Verification items for the finished model (mm, model axes). Face numbers are marked on the shaded views. Coordinates: 2 decimals unless noted, no trailing zeros. Order: outer loops, then holes, each group sorted by start corner. A loop starts at its lowest first (then second) coordinate and runs counter-clockwise, first axis right, second up.
Q1. Draft check along Z on the marked faces 1, 2, 3 and 4. Enter one of: pulls with the +Z half, pulls with the -Z half, needs draft (parallel to the pull), parting line crosses it, or undercut.
Q2. Cross-section at B-B, the plane y = -66.5. Record the boundary of the cut face in (x, z), and give its area (3 significant figures).
Q3. Cross-section at D-D, the plane z = 32. Record the boundary of the cut face in (x, y).
Q4. Cross-section at C-C, the plane x = -15.25. Record the boundary of the cut face in (y, z), and give its area (3 significant figures).
Q5. Depth check by flat-ended pin: P1, Ø3, axis at y = -26.5, z = -15, coming from the +X side; P2, Ø5.5, axis at x = -9.22, y = -50.8, coming from the -Z side. Enter the tip coordinate at first touch or a pass-through.
Q6. Thickness scan on line 1 (Z direction, x = -18.25, y = -7); line 2 (X direction, y = -39.5, z = 41); line 3 (X direction, y = -50, z = -34). Record the ranges inside material, lowest first.
Q7. Cross-section at A-A, the plane y = -50.8. Record the boundary of the cut face in (x, z).
from build123d import *

# Parameters (mm, degrees)
F1_DEPTH = 88.9
F2_R     = 3.175
F3_DEPTH = 101.6
F5_DEPTH = 3.175


with BuildPart() as f1:
    # F0 (on Front) → F1 (new body)
    with BuildSketch(Plane.XZ):
        Polygon((3.47705, 44.675883), (-21.92295, 44.675883), (-21.92295, -35.715117), (3.47705, -35.715117), (3.47705, -32.540117), (-18.74795, -32.540117), (-18.74795, 41.500883), (3.47705, 41.500883), align=None)
    extrude(amount=F1_DEPTH)

    # F2 (on face) → F3 (cut)
    with BuildSketch(Plane.XY.offset(44.675883)):
        with Locations((-9.22295, -76.2)):
            Circle(F2_R)
        with Locations((-9.22295, -50.8)):
            Circle(F2_R)
        with Locations((-9.22295, -25.4)):
            Circle(F2_R)
        with Locations((-9.22295, 0)):
            Circle(F2_R)
        with Locations((-34.62295, -76.2)):
            Circle(F2_R)
        with Locations((-34.62295, -50.8)):
            Circle(F2_R)
        with Locations((-34.62295, -25.4)):
            Circle(F2_R)
        with Locations((-34.62295, 0)):
            Circle(F2_R)
    extrude(amount=-F3_DEPTH, mode=Mode.SUBTRACT)

    # F4 (on face) → F5 (cut)
    with BuildSketch(Plane.XY.offset(44.675883)):
        with BuildLine():
            Line((-17.16045, 0), (3.47705, -11.915066))
            Line((3.47705, -11.915066), (3.47705, 0))
            Line((3.47705, 0), (-6.04795, 0))
            ThreePointArc((-6.04795, 0), (-9.22295, -3.175), (-12.39795, 0))
            Line((-12.39795, 0), (-17.16045, 0))
        make_face()
        Polygon((3.47705, -76.521958), (-17.962348, -88.9), (3.47705, -88.9), align=None)
    extrude(amount=-F5_DEPTH, mode=Mode.SUBTRACT)


solid = f1.part
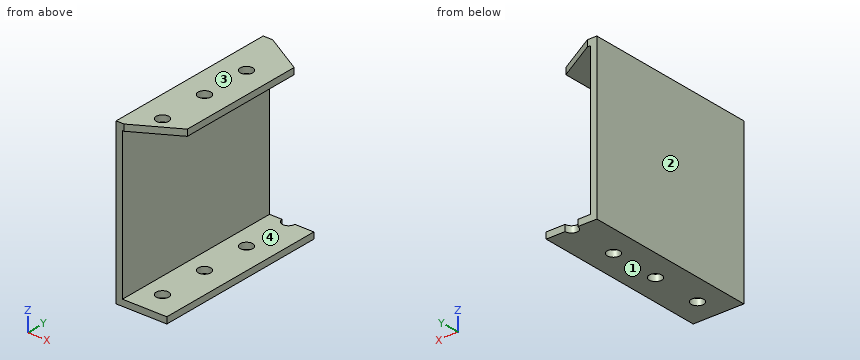
Check values:
1. face 1: pulls with the -Z half
1. face 2: needs draft
1. face 3: pulls with the +Z half
1. face 4: undercut
2. outline: (-21.92, -35.72) - (3.48, -35.72) - (3.48, -32.54) - (-18.75, -32.54) - (-18.75, 41.5) - (3.48, 41.5) - (3.48, 44.68) - (-21.92, 44.68) - close
2. area: 396 mm2
3. outline: (-21.92, -88.9) - (-18.75, -88.9) - (-18.75, 0) - (-21.92, 0) - close
4. outline: (-88.9, -35.72) - (0, -35.72) - (0, -32.54) - (-88.9, -32.54) - close; (-87.33, 41.5) - (-1.1, 41.5) - (-1.1, 44.68) - (-87.33, 44.68) - close
4. area: 556 mm2
5. P1: stops at x = -18.75
5. P2: passes through
6. line 1: z = -35.72 to -32.54, 41.5 to 44.68
6. line 2: x = -21.92 to -18.75
6. line 3: x = -21.92 to -12.3, -6.15 to 3.48
7. outline: (-21.92, -35.72) - (-12.4, -35.72) - (-12.4, -32.54) - (-18.75, -32.54) - (-18.75, 41.5) - (-12.4, 41.5) - (-12.4, 44.68) - (-21.92, 44.68) - close; (-6.05, -35.72) - (3.48, -35.72) - (3.48, -32.54) - (-6.05, -32.54) - close; (-6.05, 41.5) - (3.48, 41.5) - (3.48, 44.68) - (-6.05, 44.68) - close
